from build123d import *

# Parameters (mm, degrees)
SKETCH1_W           = 196.342
SKETCH1_H           = 50.8
BOSS_EXTRUDE1_DEPTH = 6.35
CUT_EXTRUDE1_DEPTH  = 7.62


with BuildPart() as part:
    # Sketch1 → Boss-Extrude1 (new body)
    with BuildSketch(Plane(origin=(0, 0, 0), x_dir=(1, 0, 0), z_dir=(0, 1, 0))):
        with Locations((98.171, 25.4)):
            Rectangle(SKETCH1_W, SKETCH1_H)
    extrude(amount=BOSS_EXTRUDE1_DEPTH)

    # Sketch2 → Cut-Extrude1 (cut)
    with BuildSketch(Plane.XZ):
        Polygon((136.525, -25.7175), (136.525, -36.83), (133.35, -36.83), (133.35, -11.43), (136.525, -11.43), (136.525, -22.5425), (149.225, -22.5425), (149.225, -11.43), (152.4, -11.43), (152.4, -36.83), (149.225, -36.83), (149.225, -25.7175), align=None)
    extrude(amount=-CUT_EXTRUDE1_DEPTH, mode=Mode.SUBTRACT)


solid = part.part
Design review of the part built by this model. Coordinates are the model's own, in mm. A direction names the side the tool comes from. Coordinates: 2 decimals unless noted, no trailing zeros. Write each loop counter-clockwise with the first axis right and the second up, starting at its lowest first coordinate (ties: lowest second). Pieces come first, ordered by that corner, then holes. Notation, with made-up numbers: (-25, 51.5) - (-6, 51.5) arc R23 ccw to (-6, 72.5) - close; hole circle Ø8 at (-35.5, -19.5). An arc over 180 degrees is marked (long way). One line per item, written item: value.
1) To check wall thickness, follow probe 1 along X at (y, z) = (3.25, -32) (3 decimals); probe 2 along X at (y, z) = (3.5, -23.5); probe 3 along Z at (x, y) = (140, 0.75). State the ranges of each line that lie inside material, in increasing order.
Answer sheet:
probe 1: x = 0 to 133.35, 136.525 to 149.225, 152.4 to 196.342
probe 2: x = 0 to 133.35, 152.4 to 196.34
probe 3: z = -50.8 to -25.72, -22.54 to 0
2) Insertion check: pin 1 (2 mm diameter, centred on y = 1.5, z = -39.5, fed in from -X). The pin has a flat end and moves straight along its axis. Give the tip position at first contact, or say it passes through.
Answer sheet:
pin 1: stops at x = 0
3) Add section B-B (x = 141). State the section outline as (y, z) points, plus the area to 3 significant figures.
Answer sheet:
outline: (0, -50.8) - (6.35, -50.8) - (6.35, -25.72) - (0, -25.72) - close; (0, -22.54) - (6.35, -22.54) - (6.35, 0) - (0, 0) - close
area: 302 mm2
4) Mouldability with a two-part tool opening along X and no side actions: class faces 3 (the face through (135, 3, -11.43)), 4 (the face through (97, 0, -26)), 5 (the face through (143, 3, -25.718)), 6 (the face through (0, 3, -25)) as +X half, -X half, draft (parallel to the pull), parting line (faces both ways), or undercut.
Answer sheet:
face 3: undercut
face 4: draft
face 5: undercut
face 6: -X half
5) Add section A-A (z = -30). State the section outline as (x, y) points (3 decimals).
Answer sheet:
outline: (0, 0) - (133.35, 0) - (133.35, 6.35) - (0, 6.35) - close; (136.525, 0) - (149.225, 0) - (149.225, 6.35) - (136.525, 6.35) - close; (152.4, 0) - (196.342, 0) - (196.342, 6.35) - (152.4, 6.35) - close
6) For faces 1 (the face through (97, 6.35, -26)), 2 (the face through (133.35, 3, -24)), list the 3-axis set-ups (+Z, -Z, +X, -X, +Y, -Y) from which the entire face can be reached by the end or side of a thin tool; tool diameter is ignored.
Answer sheet:
face 1: +Z, -Z, +X, -X, +Y
face 2: +Y, -Y
